Design review of the part shown in the three views and the two pictorial views. Dimensions are in mm from the part's minimum x, y and z. A direction names the side the tool comes from. Coordinates: 2 decimals unless noted, no trailing zeros. Write each loop counter-clockwise with the first axis right and the second up, starting at its lowest first coordinate (ties: lowest second). Pieces come first, ordered by that corner, then holes. Notation, with made-up numbers: (71.5, -10.5) - (75.5, -10.5) arc R19 cw to (75.5, 12.5) - close; hole circle Ø11 at (-22.5, 43.5). An arc over 180 degrees is marked (long way). Answer as CSV lines item,"result". Start each with the question number.
Q1. Clearance check with flat-ended pins moving along their axes: pin 1 (6 mm diameter, centred on x = 9.5, y = 20, fed in from -Z); pin 2 (1 mm diameter, centred on y = 12, z = 13, fed in from -X); pin 3 (1.3 mm diameter, centred on x = 30.7, z = 12.5, fed in from -Y); pin 4 (1 mm diameter, centred on y = 12.5, z = 18, fed in from +X). State where each tip first meets the part, or that it passes through.
Q2. Machinability: for the marked faces 1, 2 and 3, which of the approach directions +Z, -Z, +X, -X, +Y, -Y give a long, thin tool a straight path to every point of the face, cutting with its end or side? Answer none if there is none.
Q3. For line 1 along X through (y, z) = (5, 12.5); line 2 along Z through (x, y) = (30.7, 3); line 3 along Y through (x, z) = (28, 16.5), list the stretches that pass through material, from the lowest coordinate up. Write a range as [from, to].
Q4. We need section A-A (y = 11.75). Write out the cut boundary in (x, z).
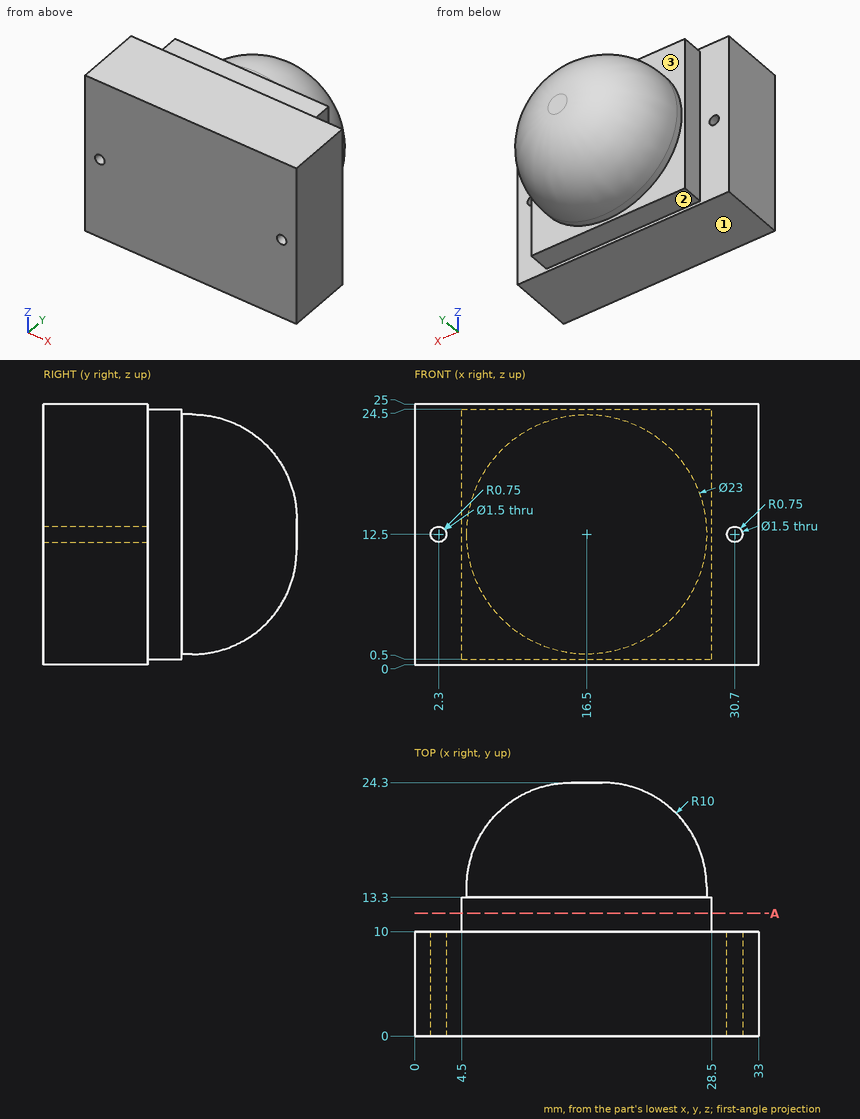
Results list:
1,pin 1,"stops at z = 2.82"
1,pin 2,"stops at x = 4.5"
1,pin 3,"passes through"
1,pin 4,"stops at x = 28.5"
2,face 1,"-Z, +X, -X, +Y, -Y"
2,face 2,"-Z, +X, -X, +Y"
2,face 3,"+Y"
3,line 1,"x = [0, 1.55], [3.05, 29.95], [31.45, 33]"
3,line 2,"z = [0, 11.75], [13.25, 25]"
3,line 3,"y = [0, 13.3]"
4,outline,"(4.5, 0.5) - (28.5, 0.5) - (28.5, 24.5) - (4.5, 24.5) - close"
